from build123d import *

# Parameters (mm, degrees)
SKETCH2_R                                         = 67.5
PALM_BASE_DEPTH                                   = 12
BOTTOM_SURFACE_REMOVED_T                          = -6
THROUGH_HOLE_FOR_FINGER_BASE_REACH                = 98.211
FINGER_BASE_CUT_OFFSET_FROM_SURFACE_REACH         = 101.211
FINGER_START                                      = -3
SKETCH4_R                                         = 64.5
SIDE_THICKNESS_CUT_DEPTH                          = 6
CSK_FOR_8_FLAT_HEAD_SOCKET_CAP_SCREW1_D           = 4.9149
CSK_FOR_8_FLAT_HEAD_SOCKET_CAP_SCREW1_CSINK_D     = 9.1186
CSK_FOR_8_FLAT_HEAD_SOCKET_CAP_SCREW1_CSINK_ANGLE = 82
SLOT_FOR_PALM_BOTTOM_REACH                        = 98.211
SLOT_FOR_PALM_BOTTOM_END_RADIUS                   = 67.5
SKETCH9_W                                         = 20
SKETCH9_H                                         = 6
SLOT_FOR_PALM_BOTTOM_DIRECTION_2_REACH            = 98.211
SLOT_FOR_PALM_BOTTOM_DIRECTION_2_END_RADIUS       = 67.5


with BuildPart() as part:
    # Sketch2 → Palm base (new body)
    with BuildSketch(Plane(origin=(0, 0, 0), x_dir=(1, 0, 0), z_dir=(0, 1, 0))):
        with Locations(Location((0, 0, 0), (0, 0, 270))):
            Circle(SKETCH2_R)
    extrude(amount=-PALM_BASE_DEPTH)

    # Bottom surface removed
    bottom_surface_removed_openings = [part.faces().sort_by_distance(p)[0] for p in [
        (0, -12, 0),
    ]]
    offset(amount=BOTTOM_SURFACE_REMOVED_T, openings=bottom_surface_removed_openings, kind=Kind.INTERSECTION)

    # Sketch3 → Through hole for finger base (cut, up to next)
    with BuildSketch(Plane(origin=(0, 0, 0), x_dir=(1, 0, 0), z_dir=(0, 1, 0)), mode=Mode.PRIVATE) as through_hole_for_finger_base_sk1:
        Polygon((25.678953914, 40.377684751), (42.53720785, 21.916935194), (26.889876526, 7.627879157), (10.031622589, 26.088628715), align=None)
    through_hole_for_finger_base_tool1 = extrude(through_hole_for_finger_base_sk1.sketch, amount=-THROUGH_HOLE_FOR_FINGER_BASE_REACH, mode=Mode.PRIVATE) & part.part
    # Sketch3 → Through hole for finger base (cut, up to next)
    with BuildSketch(Plane(origin=(0, 0, 0), x_dir=(1, 0, 0), z_dir=(0, 1, 0)), mode=Mode.PRIVATE) as through_hole_for_finger_base_sk2:
        Polygon((7.379432661, -26.959116707), (-17.139633769, -22.079016153), (-21.276006998, -42.861376859), (3.243059431, -47.741477412), align=None)
    through_hole_for_finger_base_tool2 = extrude(through_hole_for_finger_base_sk2.sketch, amount=-THROUGH_HOLE_FOR_FINGER_BASE_REACH, mode=Mode.PRIVATE) & part.part
    # Sketch3 → Through hole for finger base (cut, up to next)
    with BuildSketch(Plane(origin=(0, 0, 0), x_dir=(1, 0, 0), z_dir=(0, 1, 0)), mode=Mode.PRIVATE) as through_hole_for_finger_base_sk3:
        Polygon((-26.18008314, 9.790467137), (-23.540423594, -15.06978623), (-44.611974348, -17.307161662), (-47.251633894, 7.553091705), align=None)
    through_hole_for_finger_base_tool3 = extrude(through_hole_for_finger_base_sk3.sketch, amount=-THROUGH_HOLE_FOR_FINGER_BASE_REACH, mode=Mode.PRIVATE) & part.part
    add(through_hole_for_finger_base_tool1.solids().sort_by_distance((26.284415, 0, -24.002782))[0], mode=Mode.SUBTRACT)
    add(through_hole_for_finger_base_tool2.solids().sort_by_distance((-6.948287, 0, 34.910247))[0], mode=Mode.SUBTRACT)
    add(through_hole_for_finger_base_tool3.solids().sort_by_distance((-35.396029, 0, 3.758347))[0], mode=Mode.SUBTRACT)

    # Sketch7 → Finger base cut offset from surface (cut, up to next)
    with BuildSketch(Plane(origin=(0, 0, 0), x_dir=(1, 0, 0), z_dir=(0, 1, 0)).offset(FINGER_START), mode=Mode.PRIVATE) as finger_base_cut_offset_from_surface_sk1:
        Polygon((8.179769152, -22.937989812), (-16.339297278, -18.057889258), (-17.139633769, -22.079016153), (7.379432661, -26.959116707), align=None)
    finger_base_cut_offset_from_surface_tool1 = extrude(finger_base_cut_offset_from_surface_sk1.sketch, amount=-FINGER_BASE_CUT_OFFSET_FROM_SURFACE_REACH, mode=Mode.PRIVATE) & part.part
    # Sketch7 → Finger base cut offset from surface (cut, up to next)
    with BuildSketch(Plane(origin=(0, 0, 0), x_dir=(1, 0, 0), z_dir=(0, 1, 0)).offset(FINGER_START), mode=Mode.PRIVATE) as finger_base_cut_offset_from_surface_sk2:
        Polygon((-22.076343489, -46.882503753), (2.442722941, -51.762604307), (3.243059431, -47.741477412), (-21.276006998, -42.861376859), align=None)
    finger_base_cut_offset_from_surface_tool2 = extrude(finger_base_cut_offset_from_surface_sk2.sketch, amount=-FINGER_BASE_CUT_OFFSET_FROM_SURFACE_REACH, mode=Mode.PRIVATE) & part.part
    # Sketch7 → Finger base cut offset from surface (cut, up to next)
    with BuildSketch(Plane(origin=(0, 0, 0), x_dir=(1, 0, 0), z_dir=(0, 1, 0)).offset(FINGER_START), mode=Mode.PRIVATE) as finger_base_cut_offset_from_surface_sk3:
        Polygon((10.031622589, 26.088628715), (7.004059662, 23.323875069), (23.862313598, 4.863125512), (26.889876526, 7.627879157), align=None)
    finger_base_cut_offset_from_surface_tool3 = extrude(finger_base_cut_offset_from_surface_sk3.sketch, amount=-FINGER_BASE_CUT_OFFSET_FROM_SURFACE_REACH, mode=Mode.PRIVATE) & part.part
    # Sketch7 → Finger base cut offset from surface (cut, up to next)
    with BuildSketch(Plane(origin=(0, 0, 0), x_dir=(1, 0, 0), z_dir=(0, 1, 0)).offset(FINGER_START), mode=Mode.PRIVATE) as finger_base_cut_offset_from_surface_sk4:
        Polygon((45.564770778, 24.681688839), (42.53720785, 21.916935194), (25.678953914, 40.377684751), (28.706516842, 43.142438397), align=None)
    finger_base_cut_offset_from_surface_tool4 = extrude(finger_base_cut_offset_from_surface_sk4.sketch, amount=-FINGER_BASE_CUT_OFFSET_FROM_SURFACE_REACH, mode=Mode.PRIVATE) & part.part
    # Sketch7 → Finger base cut offset from surface (cut, up to next)
    with BuildSketch(Plane(origin=(0, 0, 0), x_dir=(1, 0, 0), z_dir=(0, 1, 0)).offset(FINGER_START), mode=Mode.PRIVATE) as finger_base_cut_offset_from_surface_sk5:
        Polygon((-48.6890559, -17.740065828), (-44.611974348, -17.307161662), (-47.251633894, 7.553091705), (-51.328715447, 7.120187539), align=None)
    finger_base_cut_offset_from_surface_tool5 = extrude(finger_base_cut_offset_from_surface_sk5.sketch, amount=-FINGER_BASE_CUT_OFFSET_FROM_SURFACE_REACH, mode=Mode.PRIVATE) & part.part
    # Sketch7 → Finger base cut offset from surface (cut, up to next)
    with BuildSketch(Plane(origin=(0, 0, 0), x_dir=(1, 0, 0), z_dir=(0, 1, 0)).offset(FINGER_START), mode=Mode.PRIVATE) as finger_base_cut_offset_from_surface_sk6:
        Polygon((-23.540423594, -15.06978623), (-26.18008314, 9.790467137), (-22.103001588, 10.223371302), (-19.463342042, -14.636882065), align=None)
    finger_base_cut_offset_from_surface_tool6 = extrude(finger_base_cut_offset_from_surface_sk6.sketch, amount=-FINGER_BASE_CUT_OFFSET_FROM_SURFACE_REACH, mode=Mode.PRIVATE) & part.part
    add(finger_base_cut_offset_from_surface_tool1.solids().sort_by_distance((-4.479932, -3, 22.508503))[0], mode=Mode.SUBTRACT)
    add(finger_base_cut_offset_from_surface_tool2.solids().sort_by_distance((-9.416642, -3, 47.311991))[0], mode=Mode.SUBTRACT)
    add(finger_base_cut_offset_from_surface_tool3.solids().sort_by_distance((16.946968, -3, -15.475877))[0], mode=Mode.SUBTRACT)
    add(finger_base_cut_offset_from_surface_tool4.solids().sort_by_distance((35.621862, -3, -32.529687))[0], mode=Mode.SUBTRACT)
    add(finger_base_cut_offset_from_surface_tool5.solids().sort_by_distance((-47.970345, -3, 5.093487))[0], mode=Mode.SUBTRACT)
    add(finger_base_cut_offset_from_surface_tool6.solids().sort_by_distance((-22.821713, -3, 2.423207))[0], mode=Mode.SUBTRACT)

    # Sketch4 → Side thickness cut (cut)
    with BuildSketch(Plane.XZ.offset(12)):
        with Locations(Location((0, 0, 0), (0, 0, 270))):
            Circle(SKETCH4_R)
    extrude(amount=-SIDE_THICKNESS_CUT_DEPTH, mode=Mode.SUBTRACT)

    # CSK for #8 Flat Head Socket Cap Screw1 (through all)
    with Locations(Plane(origin=(-32.5, 0, -50.435602505), x_dir=(0, 0, 1), z_dir=(0, 1, 0))):
        with Locations((0, 0), (0, 65), (100.87120501, 65), (100.87120501, 0)):
            CounterSinkHole(CSK_FOR_8_FLAT_HEAD_SOCKET_CAP_SCREW1_D / 2, CSK_FOR_8_FLAT_HEAD_SOCKET_CAP_SCREW1_CSINK_D / 2, counter_sink_angle=CSK_FOR_8_FLAT_HEAD_SOCKET_CAP_SCREW1_CSINK_ANGLE)

    # Slot for palm bottom: up to this cylinder (the profile starts inside it)
    slot_for_palm_bottom_end = Plane(origin=(0, -9, 0), z_dir=(0, 1, 0)) * Cylinder(SLOT_FOR_PALM_BOTTOM_END_RADIUS, 332.422, mode=Mode.PRIVATE)
    # Sketch9 → Slot for palm bottom (cut, up to the surface)
    with BuildSketch(Plane(origin=(0, 0, 0), x_dir=(0, 0, -1), z_dir=(1, 0, 0)), mode=Mode.PRIVATE) as slot_for_palm_bottom_sk1:
        with Locations((0, -9)):
            Rectangle(SKETCH9_W, SKETCH9_H)
    slot_for_palm_bottom_tool1 = extrude(slot_for_palm_bottom_sk1.sketch, amount=-SLOT_FOR_PALM_BOTTOM_REACH, mode=Mode.PRIVATE) & slot_for_palm_bottom_end
    add(slot_for_palm_bottom_tool1.solids().sort_by_distance((0, -9, 0))[0], mode=Mode.SUBTRACT)

    # Slot for palm bottom direction 2: up to this cylinder (the profile starts inside it)
    slot_for_palm_bottom_direction_2_end = Plane(origin=(0, -9, 0), z_dir=(0, 1, 0)) * Cylinder(SLOT_FOR_PALM_BOTTOM_DIRECTION_2_END_RADIUS, 332.422, mode=Mode.PRIVATE)
    # Sketch9 → Slot for palm bottom direction 2 (cut, up to the surface)
    with BuildSketch(Plane(origin=(0, 0, 0), x_dir=(0, 0, -1), z_dir=(1, 0, 0)), mode=Mode.PRIVATE) as slot_for_palm_bottom_direction_2_sk1:
        with Locations((0, -9)):
            Rectangle(SKETCH9_W, SKETCH9_H)
    slot_for_palm_bottom_direction_2_tool1 = extrude(slot_for_palm_bottom_direction_2_sk1.sketch, amount=SLOT_FOR_PALM_BOTTOM_DIRECTION_2_REACH, mode=Mode.PRIVATE) & slot_for_palm_bottom_direction_2_end
    add(slot_for_palm_bottom_direction_2_tool1.solids().sort_by_distance((0, -9, 0))[0], mode=Mode.SUBTRACT)


solid = part.part
Check sheet for the modelled part. Datum: model origin and axes. Units: mm. A direction names the side the tool comes from. Round coordinates to 2 decimals unless told otherwise and drop trailing zeros. Order: outer loops, then holes, each group sorted by start corner. A loop starts at its lowest first (then second) coordinate and runs counter-clockwise, first axis right, second up.
(1) Cross-section at C-C, the plane x = 32.5. Enter the section's corners in (y, z).
(2) Draft check along X on faces 1 (the flat face through (17, -3, -15)), 2 (the flat face through (36, -3, -33)), 3 (the flat face through (0, -12, 66)). Enter one of: pulls with the +X half, pulls with the -X half, needs draft (parallel to the pull), parting line crosses it, or undercut.
(3) Cross-section at B-B, the plane z = 0. Enter the section's corners in (x, y).
(4) Cross-section at D-D, the plane x = 49. Enter the section's corners in (y, z), and give its area (3 significant figures).
(5) Go/stop test with flat-tipped pins: P1, Ø1, axis at y = -6, z = 45, coming from the +X side; P2, Ø3, axis at x = 34.5, y = -3, coming from the +Z side; P3, Ø2.5, axis at x = 0.5, z = 20.5, coming from the -Y side; P4, Ø3, axis at x = 32.5, z = -50.44, coming from the +Y side. Record where each tip stops, or that it passes through.
(6) Access from +Z, -Z, +X, -X, +Y, -Y to the whole of each face (thin tool, end or side, straight path). Record for faces 4 (the flat face through (-65, -9, -10)), 5 (the flat face through (-24.88, -1.48, 2.47)), 6 (the conical face through (35.04, -2.3, 50.77)), 7 (the flat face through (-9.99, -4.48, 49.29)), 8 (the flat face through (5.26, -12, -64.44)).
(7) Scan lines: probe 1 along Z at (x, y) = (32.5, -4.95); probe 2 along Z at (x, y) = (-1, -8.5); probe 3 along Z at (x, y) = (-32.5, -4.75). Record each from-to range of solid material in increasing order.
(8) Cross-section at A-A, the plane x = 0. Enter the section's corners in (y, z), and give its area (3 significant figures).
Check sheet entries:
1. outline: (-12, -59.16) - (0, -59.16) - (0, -54.99) - (-2.42, -52.89) - (-6, -52.89) - (-6, -55.71) - (-12, -55.71) - close; (-12, 55.71) - (-6, 55.71) - (-6, 52.89) - (-2.42, 52.89) - (0, 54.99) - (0, 59.16) - (-12, 59.16) - close; (-6, -47.98) - (-2.42, -47.98) - (0, -45.88) - (0, -32.91) - (-3, -32.91) - (-3, -38.99) - (-6, -38.99) - close; (-6, -12.75) - (0, -12.75) - (0, 45.88) - (-2.42, 47.98) - (-6, 47.98) - close
2. face 1: undercut
2. face 2: undercut
2. face 3: needs draft
3. outline: (-67.5, -6) - (-50.57, -6) - (-50.57, -3) - (-46.45, -3) - (-46.45, 0) - (-67.5, 0) - close; (-25.14, -3) - (-21.02, -3) - (-21.02, -6) - (67.5, -6) - (67.5, 0) - (-25.14, 0) - close
4. outline: (-12, -46.42) - (0, -46.42) - (0, 46.42) - (-12, 46.42) - (-12, 41.94) - (-6, 41.94) - (-6, -41.94) - (-12, -41.94) - close
4. area: 611 mm2
5. P1: stops at x = 50.75
5. P2: stops at z = 58.88
5. P3: stops at y = -6
5. P4: passes through
6. face 4: +X, -X, -Y
6. face 5: +Y, -Y
6. face 6: +Y
6. face 7: -Y
6. face 8: +Z, -Z, +X, -X, -Y
7. probe 1: z = -59.16 to -52.89, -47.98 to -38.99, -12.75 to 47.98, 52.89 to 59.16
7. probe 2: z = -67.49 to -64.49, 64.49 to 67.49
7. probe 3: z = -59.16 to -52.89, -47.98 to -9.12, 16.02 to 47.98, 52.89 to 59.16
8. outline: (-12, -67.5) - (0, -67.5) - (0, 25.49) - (-3, 25.49) - (-3, 21.31) - (-6, 21.31) - (-6, -64.5) - (-12, -64.5) - close; (-12, 64.5) - (-6, 64.5) - (-6, 51.28) - (-3, 51.28) - (-3, 47.1) - (0, 47.1) - (0, 67.5) - (-12, 67.5) - close
8. area: 691 mm2
